The figure shows three views and two pictorial views of one solid part (mm, origin at its lowest corner). Answer the questions. A direction names the side the tool comes from. Coordinates: 2 decimals unless noted, no trailing zeros. Loops run counter-clockwise (first coordinate to the right, second up) from the corner with the lowest first, then second, coordinate; pieces in that order, holes last. Notation, with made-up numbers: (88.5, 10.5) -> (123.5, 10.5) arc R26 ccw to (123.5, 47.5) -> close; hole circle Ø10 at (78, 54.25). An arc over 180 degrees is marked (long way). Answer as a JSON object with one key per item and string values. Group by question number.
1) Flat-ended cylindrical pins translate along their axes: P1, Ø1.5, axis at x = 26.5, z = 6, coming from the -Y side (3 decimals); P2, Ø2, axis at x = 8.5, y = 5, coming from the +Z side. Find the tip coordinate at first contact, or state that the pin passes through.
2) Section A-A, the plane y = 12.5 is taken. Give the vertices of the cut face in (x, z), plus the area to 3 significant figures.
3) Determine the mould class of the marked faces 1, 2 and 3 for opening direction Y: released by +Y, released by -Y, zero draft, split by the parting line, or undercut.
4) Which of the six approach directions +Z, -Z, +X, -X, +Y, -Y give full straight-line access (tool end or side, diameter ignored) to the marked faces 4, 5 and 6?
5) Section B-B, the plane z = 2.75 is taken. Give the vertices of the cut face in (x, y), plus the area to 3 significant figures.
6) Consider probe 1 along X at (y, z) = (14.25, 7); probe 2 along X at (y, z) = (14, 6) (1 decimal); probe 3 along Z at (x, y) = (43, 16.75). Determine where each line is inside the solid, lowest interval first. Write a range as [from, to].
7) Section C-C, the plane x = 6 is taken. Give the vertices of the cut face in (y, z) (1 decimal).
8) Section D-D, the plane x = 17 is taken. Give the vertices of the cut face in (y, z) (1 decimal), plus the area to 3 significant figures.
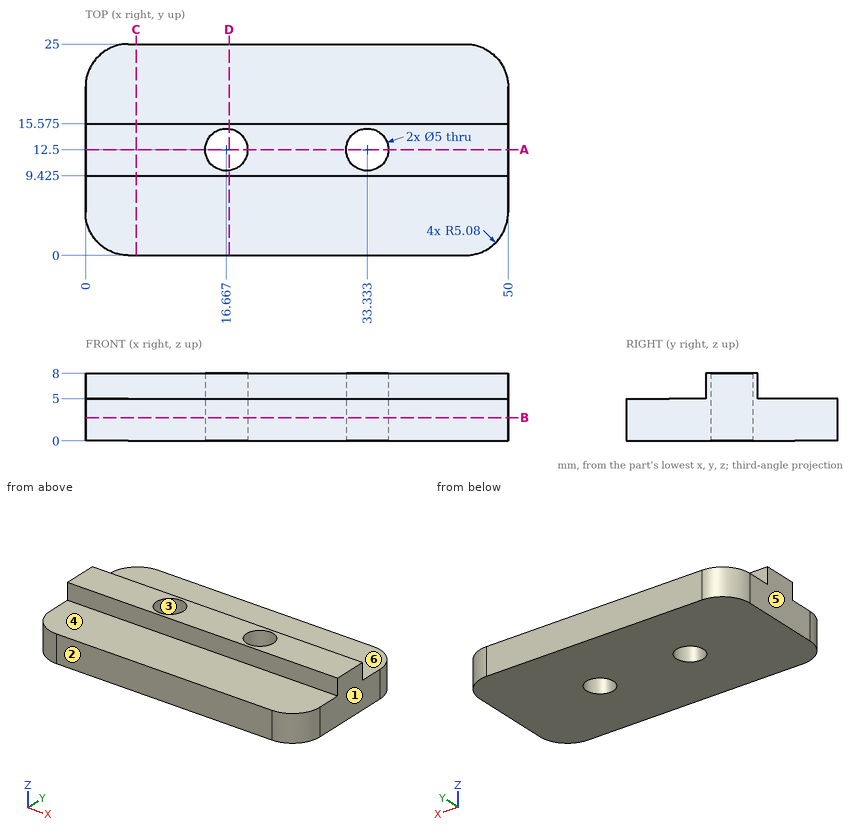
Determined:
{
 "1": {"P1": "y = 9.425", "P2": "z = 5"},
 "2": {"outline": "(0, 0) -> (14.17, 0) -> (14.17, 8) -> (0, 8) -> close; (19.17, 0) -> (30.83, 0) -> (30.83, 8) -> (19.17, 8) -> close; (35.83, 0) -> (50, 0) -> (50, 8) -> (35.83, 8) -> close", "area": "320 mm²"},
 "3": {"face 1": "zero draft", "face 2": "released by -Y", "face 3": "undercut"},
 "4": {"face 4": "+Z, +X, -X, -Y", "face 5": "+Z, -Z, -X, +Y, -Y", "face 6": "+Z, +X, -X, +Y"},
 "5": {"outline": "(0, 5.08) arc R5.08 ccw to (5.08, 0) -> (44.92, 0) arc R5.08 ccw to (50, 5.08) -> (50, 19.92) arc R5.08 ccw to (44.92, 25) -> (5.08, 25) arc R5.08 ccw to (0, 19.92) -> close; hole circle Ø5 at (16.67, 12.5); hole circle Ø5 at (33.33, 12.5)", "area": "1,190 mm²"},
 "6": {"probe 1": "[0, 14.88], [18.45, 31.55], [35.12, 50]", "probe 2": "[0, 14.7], [18.7, 31.3], [35.3, 50]", "probe 3": "[0, 5]"},
 "7": {"outline": "(0, 0) -> (25, 0) -> (25, 5) -> (15.6, 5) -> (15.6, 8) -> (9.4, 8) -> (9.4, 5) -> (0, 5) -> close"},
 "8": {"outline": "(0, 0) -> (10, 0) -> (10, 8) -> (9.4, 8) -> (9.4, 5) -> (0, 5) -> close; (15, 0) -> (25, 0) -> (25, 5) -> (15.6, 5) -> (15.6, 8) -> (15, 8) -> close", "area": "104 mm²"}
}
